```python
from build123d import *

# Parameters (mm, degrees)
SKETCH1_W              = 25.4
SKETCH1_H              = 50.8
SKETCH1_R              = 2.413
SKETCH1_R_2            = 2.38125
BOSS_EXTRUDE1_DEPTH    = 3.175
SKETCH2_W              = 25.4
SKETCH2_H              = 3.175
BOSS_EXTRUDE2_DEPTH    = 44.45
SKETCH3_R              = 2.413
CUT_EXTRUDE1_DEPTH     = 44.45
FILLET1_R              = 2.54
CONVERT_SOLID1_START   = -12.7
CONVERT_SOLID1_DEPTH   = 25.4
CONVERT_SOLID1_2_DEPTH = 25.4


# Read off the part's stored shape, not the designer's step: Convert-Solid1
with BuildPart() as part:
    # Sketch1 → Boss-Extrude1 (new body)
    with BuildSketch(Plane.XY):
        Rectangle(SKETCH1_W, SKETCH1_H)
        with Locations((0, 12.7)):
            Circle(SKETCH1_R, mode=Mode.SUBTRACT)
        with Locations((0.348627451, 0)):
            Circle(SKETCH1_R, mode=Mode.SUBTRACT)
        with Locations((0.348627451, -12.7)):
            Circle(SKETCH1_R_2, mode=Mode.SUBTRACT)
    extrude(amount=BOSS_EXTRUDE1_DEPTH)

    # Sketch2 → Boss-Extrude2 (add)
    with BuildSketch(Plane.XY.offset(3.175)):
        with Locations((0, 23.8125)):
            Rectangle(SKETCH2_W, SKETCH2_H)
    extrude(amount=BOSS_EXTRUDE2_DEPTH)

    # Sketch3 → Cut-Extrude1 (cut)
    with BuildSketch(Plane(origin=(0, 25.4, 0), x_dir=(1, 0, 0), z_dir=(0, 1, 0))):
        with Locations(Location((0, -12.7, 0), (0, 0, 270))):
            Circle(SKETCH3_R)
        with Locations(Location((0, -25.4, 0), (0, 0, 270))):
            Circle(SKETCH3_R)
        with Locations(Location((0, -38.1, 0), (0, 0, 270))):
            Circle(SKETCH3_R)
    extrude(amount=-CUT_EXTRUDE1_DEPTH, mode=Mode.SUBTRACT)

    # Fillet1
    fillet1_edges = [part.edges().sort_by_distance(p)[0] for p in [
        (-12.7, 23.8125, 47.625),
        (12.7, 23.8125, 47.625),
        (12.7, -25.4, 1.5875),
        (-12.7, -25.4, 1.5875),
    ]]
    fillet(fillet1_edges, radius=FILLET1_R)

    # Convert-Solid1 outline → Convert-Solid1 (cut)
    with BuildSketch(Plane.YZ.offset(CONVERT_SOLID1_START)):
        with BuildLine():
            Line((25.4, 0), (25.4, 5.555000066))
            ThreePointArc((25.4, 5.555000066), (23.77297815, 1.62702185), (19.844999934, 0))
            Line((19.844999934, 0), (25.4, 0))
        make_face()
    extrude(amount=CONVERT_SOLID1_DEPTH, mode=Mode.SUBTRACT)

    # Convert-Solid1 2 outline → Convert-Solid1 2 (add)
    with BuildSketch(Plane.YZ.offset(CONVERT_SOLID1_START)):
        with BuildLine():
            Line((22.225, 3.175), (22.225, 5.555000066))
            ThreePointArc((22.225, 5.555000066), (21.52791412, 3.87208588), (19.844999934, 3.175))
            Line((19.844999934, 3.175), (22.225, 3.175))
        make_face()
    extrude(amount=CONVERT_SOLID1_2_DEPTH)


solid = part.part
```
Here's how the part is built. I have some questions about the finished solid (model axes, mm). A direction names the side the tool comes from. Coordinates: 2 decimals unless noted, no trailing zeros. Loops run counter-clockwise (first coordinate to the right, second up) from the corner with the lowest first, then second, coordinate; pieces in that order, holes last. Notation, with made-up numbers: M 71,68 L 113,68 A17 ccw 113,77 Z; hole C -38,-17 d4. An arc over 180 degrees is marked long. One line per item, written item: value.
1. On a 3-axis mill with a long thin cutter (end or side, diameter ignored), from which of +Z, -Z, +X, -X, +Y, -Y can I reach the whole of each face in a straight line? I mean faces 1 (the flat face through (3, 22.225, 26)), 2 (the cylindrical face through (-0.178, 23.816, 1.67)). Say none if no direction works.
Geometry says:
face 1: +Z, +X, -X, -Y
face 2: -Z, +X, -X, +Y
2. Imagine slicing it at D-D (z = 19.5). List the corners of the cut face in (x, y) for me (3 decimals).
Geometry says:
outline: M -12.7,22.225 L 12.7,22.225 L 12.7,25.4 L -12.7,25.4 Z
3. Imagine slicing it at C-C (x = -3.5). List the corners of the cut face in (y, z) for me (3 decimals).
Geometry says:
outline: M -25.4,0 L 19.845,0 A5.555 ccw 25.4,5.555 L 25.4,47.625 L 22.225,47.625 L 22.225,5.555 A2.38 cw 19.845,3.175 L -25.4,3.175 Z
4. Thinking about a two-plate mould opening in X: for faces 3 (the flat face through (-3, -2, 3.175)), 4 (the flat face through (12.7, 10, 3)), 5 (the cylindrical face through (-0.523, 10.344, 1.565)), which applies, +X half, -X half, draft (parallel to the pull), parting line (faces both ways), or undercut?
Geometry says:
face 3: draft
face 4: +X half
face 5: undercut
5. Imagine slicing it at B-B (z = 12.7). List the corners of the cut face in (x, y) for me (3 decimals), and give its area (3 significant figures).
Geometry says:
outline: M -12.7,22.225 L -2.413,22.225 L -2.413,25.4 L -12.7,25.4 Z; M 2.413,22.225 L 12.7,22.225 L 12.7,25.4 L 2.413,25.4 Z
area: 65.3 mm2
6. Will these pins go through, and if not, where does the flat tip stop? pin 1 Ø6.5 at (x, y) = (0.35, 0) entering from +Z (3 decimals); pin 2 Ø6.5 at (x, z) = (0, 38.1) entering from +Y; pin 3 Ø3 at (x, y) = (0.35, -12.7) entering from +Z; pin 4 Ø7.5 at (x, z) = (-6, 32.5) entering from -Y (3 decimals).
Geometry says:
pin 1: stops at z = 3.175
pin 2: stops at y = 25.4
pin 3: passes through
pin 4: stops at y = 22.225
7. Please list where these lines run through material, in increasing order: probe 1 along X at (y, z) = (23.55, 25.4); probe 2 along Z at (x, y) = (9, -3.5) (3 decimals); probe 3 along X at (y, z) = (14, 2.5).
Geometry says:
probe 1: x = -12.7 to -2.41, 2.41 to 12.7
probe 2: z = 0 to 3.175
probe 3: x = -12.7 to -2.03, 2.03 to 12.7
8. Imagine slicing it at A-A (y = 0). List the corners of the cut face in (x, z) for me (3 decimals).
Geometry says:
outline: M -12.7,0 L -2.064,0 L -2.064,3.175 L -12.7,3.175 Z; M 2.762,0 L 12.7,0 L 12.7,3.175 L 2.762,3.175 Z
